Autodesk Inventor part; units mm, degrees
ref_plane "YZ Plane" through (0, 0, 0) normal (1, 0, 0) x (0, 1, 0)
ref_plane "XZ Plane" through (0, 0, 0) normal (0, 1, 0) x (-1, 0, 0)
ref_plane "XY Plane" through (0, 0, 0) normal (0, 0, 1) x (1, 0, 0)
sketch "Sketch1" plane through (0, 0, 0) normal (1, 0, 0) x (0, 1, 0)
  line L0 (22.225, 15.875) -> (-22.225, 15.875)
  line L1 (-22.225, 15.875) -> (-22.225, -15.875)
  line L2 (-22.225, -15.875) -> (22.225, -15.875)
  line L3 (22.225, -15.875) -> (22.225, 15.875)
  line L4 (22.225, 15.875) -> (-22.225, -15.875) construction
  line L5 (-22.225, 15.875) -> (22.225, -15.875) construction
  line L6 (15.875, 9.525) -> (-15.875, 9.525) construction
  line L7 (-15.875, 9.525) -> (-15.875, -9.525) construction
  line L8 (-15.875, -9.525) -> (15.875, -9.525) construction
  line L9 (15.875, -9.525) -> (15.875, 9.525) construction
  line L10 (15.875, 9.525) -> (-15.875, -9.525) construction
  line L11 (-15.875, 9.525) -> (15.875, -9.525) construction
  point P0 (0, 0)
  dimension "d0" = 44.45
  dimension "d1" = 31.75
  dimension "d2" = 31.75
  dimension "d3" = 19.05
extrude "Extrusion1" add sketch "Sketch1" along normal blind 6.35
hole "Hole1" at (0, 15.875, 9.525) at (0, 15.875, -9.525) at (0, -15.875, 9.525) at (0, -15.875, -9.525) direction (1, 0, 0) diameter 5.1054 end through all
sketch "Sketch2" plane through (6.35, 0, 0) normal (1, 0, 0) x (0, 0, -1)
  line L0 (3.8812, 6.35) -> (-3.8812, -6.35) construction
  point P0 (0, 0)
  point P1 (0, 0)
  dimension "d13" = 14.8844
  dimension "d27" = 6.35
hole "Hole2" at (6.35, 6.35, -3.8812) at (6.35, -6.35, 3.8812) direction (-1, 0, 0) diameter 1.9406 end through all
sketch "Sketch3" plane through (6.35, 0, 0) normal (1, 0, 0) x (0, 0, -1)
  circle A0 centre (0, 0) radius 3.81
  dimension "d21" = 7.62
extrude "Extrusion2" cut sketch "Sketch3" against normal blind 6.35
fillet "Fillet1" radius 3.175 4 edges at (3.175, 22.225, 15.875) (3.175, 22.225, -15.875) (3.175, -22.225, -15.875) (3.175, -22.225, 15.875)
properties part number "AR-015" material "ABS Plastic"
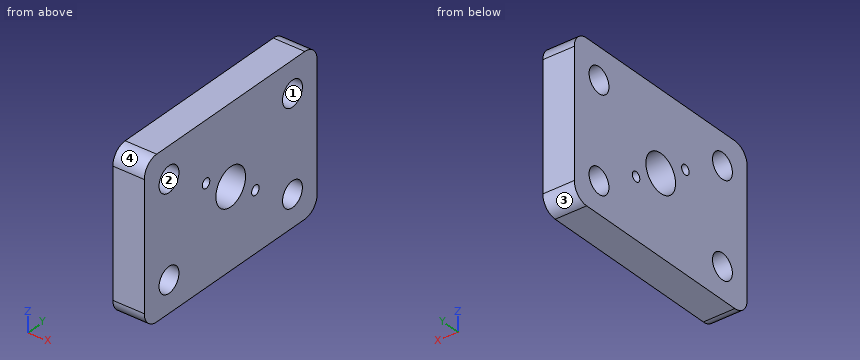
Model file for the job. Use its own axes, mm. Face numbers are marked on the shaded views. Coordinates: 2 decimals unless noted, no trailing zeros. Order: outer loops, then holes, each group sorted by start corner. A loop starts at its lowest first (then second) coordinate and runs counter-clockwise, first axis right, second up. Notation, with made-up numbers: (35.25, 17) -> (40.25, 17) arc R18 ccw to (40.25, 23) -> close; hole circle Ø11 at (82.5, 85). An arc over 180 degrees is marked (long way). Return JSON: item names as keys, results as strings.
Item 1: Slice it at B-B (x = 2.5). Count the separate pieces of the cut face and the enclosed holes in it, then the cut area to 3 significant figures.
Model answer:
{"separate pieces": "1", "enclosed holes": "7", "area": "1,270 mm²"}
Item 2: Slice it at A-A (z = 0). Write the cut outline in (x, y) (3 decimals), then the cut area to 3 significant figures.
Model answer:
{"outline": "(0, -22.225) -> (6.35, -22.225) -> (6.35, -3.81) -> (0, -3.81) -> close; (0, 3.81) -> (6.35, 3.81) -> (6.35, 22.225) -> (0, 22.225) -> close", "area": "234 mm²"}
Item 3: Slice it at D-D (y = 16.5). Write the cut outline in (x, z) (3 decimals), then the cut area to 3 significant figures.
Model answer:
{"outline": "(0, -15.875) -> (6.35, -15.875) -> (6.35, -12) -> (0, -12) -> close; (0, -7.05) -> (6.35, -7.05) -> (6.35, 7.05) -> (0, 7.05) -> close; (0, 12) -> (6.35, 12) -> (6.35, 15.875) -> (0, 15.875) -> close", "area": "139 mm²"}
Item 4: Mould opens along Z. For the marked faces 1, 2, 3 and 4 say: pulls with the +Z half, pulls with the -Z half, needs draft (parallel to the pull), parting line crosses it, or undercut.
Model answer:
{"face 1": "undercut", "face 2": "undercut", "face 3": "pulls with the -Z half", "face 4": "pulls with the +Z half"}
Item 5: Slice it at C-C (y = 0). Write the cut outline in (x, z) (3 decimals), then the cut area to 3 significant figures.
Model answer:
{"outline": "(0, -15.875) -> (6.35, -15.875) -> (6.35, -3.81) -> (0, -3.81) -> close; (0, 3.81) -> (6.35, 3.81) -> (6.35, 15.875) -> (0, 15.875) -> close", "area": "153 mm²"}
Item 6: Wall check: line 1 along Z through (x, y) = (5.5, 16) (3 decimals); line 2 along Y through (x, z) = (3.75, -9) (3 decimals); line 3 along Y through (x, z) = (2.5, 11) (3 decimals). Give the ranges that are in metal, low to high. Write a range as from..to.
Model answer:
{"line 1": "z = -15.875..-12.075, -6.975..6.975, 12.075..15.875", "line 2": "y = -22.225..-18.373, -13.377..13.377, 18.373..22.225", "line 3": "y = -22.225..-17.958, -13.792..13.792, 17.958..22.225"}
